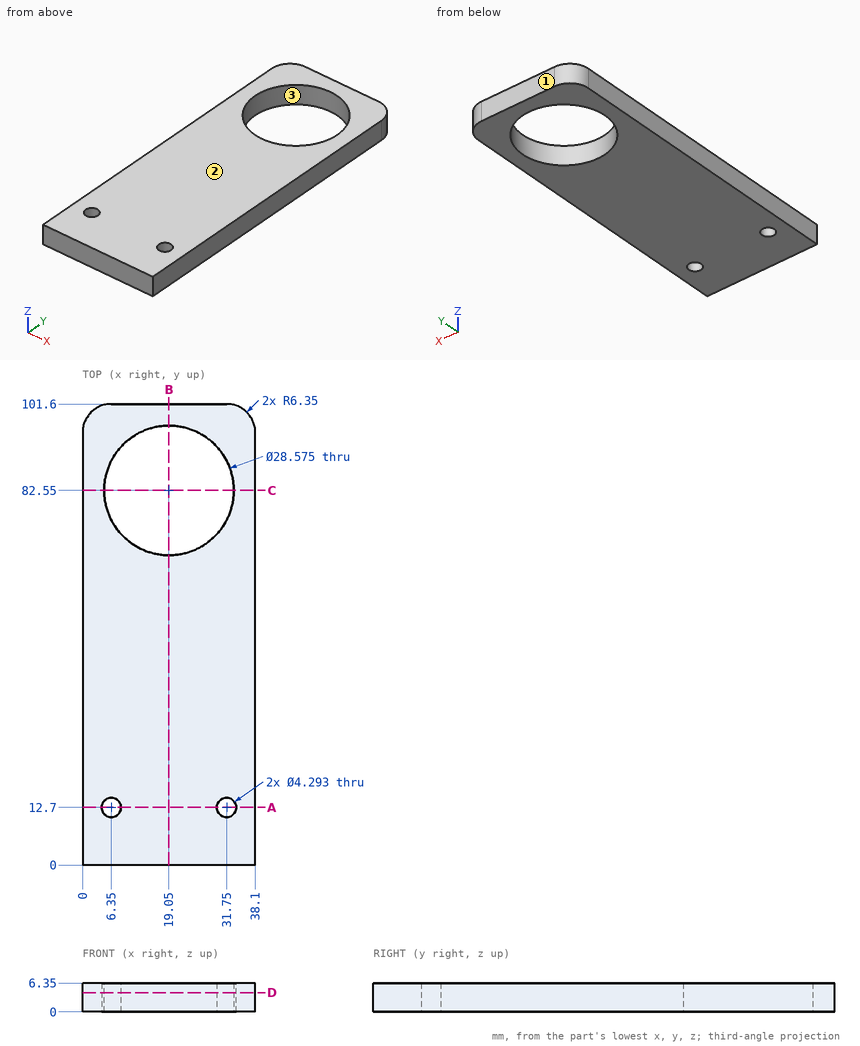
The drawing under review shows one solid part. Ordinate dimensions are in mm from its lowest x, y, z. Give positions to 0.01 mm unless a question says otherwise; leave off trailing zeros. Write each loop counter-clockwise with the first axis right and the second up, starting at its lowest first coordinate (ties: lowest second). Pieces come first, ordered by that corner, then holes. Notation, with made-up numbers: (-7, -24.5) -> (37, -24.5) arc R9 cw to (37, -12.5) -> close; hole circle Ø7 at (65.5, 0.25). An arc over 180 degrees is marked (long way). Answer in a Markdown table with one row per item.
(1) Consider section B-B (x = 19.05). State the section outline as (y, z) points, then the cut area to 3 significant figures.
Results:
| item | result |
|---|---|
| outline | (0, 0) -> (68.26, 0) -> (68.26, 6.35) -> (0, 6.35) -> close; (96.84, 0) -> (101.6, 0) -> (101.6, 6.35) -> (96.84, 6.35) -> close |
| area | 464 mm2 |
(2) Consider section A-A (y = 12.7). State the section outline as (x, z) points.
Results:
| item | result |
|---|---|
| outline | (0, 0) -> (4.2, 0) -> (4.2, 6.35) -> (0, 6.35) -> close; (8.5, 0) -> (29.6, 0) -> (29.6, 6.35) -> (8.5, 6.35) -> close; (33.9, 0) -> (38.1, 0) -> (38.1, 6.35) -> (33.9, 6.35) -> close |
(3) Consider section C-C (y = 82.55). State the section outline as (x, z) points.
Results:
| item | result |
|---|---|
| outline | (0, 0) -> (4.76, 0) -> (4.76, 6.35) -> (0, 6.35) -> close; (33.34, 0) -> (38.1, 0) -> (38.1, 6.35) -> (33.34, 6.35) -> close |
(4) Mouldability with a two-part tool opening along Y and no side actions: class the marked faces 1, 2 and 3 as +Y half, -Y half, draft (parallel to the pull), parting line (faces both ways), or undercut.
Results:
| item | result |
|---|---|
| face 1 | +Y half |
| face 2 | draft |
| face 3 | undercut |
(5) To check wall thickness, follow probe 1 along X at (y, z) = (12.7, 3.5); probe 2 along Y at (x, z) = (19, 5.5); probe 3 along Y at (x, z) = (6.5, 5) (1 decimal). State the ranges of each line that lie inside material, in increasing order.
Results:
| item | result |
|---|---|
| probe 1 | 0 to 4.2, 8.5 to 29.6, 33.9 to 38.1 |
| probe 2 | 0 to 68.26, 96.84 to 101.6 |
| probe 3 | 0 to 10.6, 14.8 to 75.7, 89.4 to 101.6 |
(6) Consider section D-D (z = 4.25). Count the separate pieces of the cut face and the enclosed holes in it, then the cut area to 3 significant figures.
Results:
| item | result |
|---|---|
| separate pieces | 1 |
| enclosed holes | 3 |
| area | 3,180 mm2 |
